```python
from build123d import *

# Parameters (mm, degrees)
F0_W     = 100.2733111382
F0_H     = 50.1366546378
F1_DEPTH = 50
F2_W     = 90.2733111382
F2_H     = 8.7347067715
F3_DEPTH = 50.001
F5_W     = 40.5144635588
F5_H     = 41.020902805
F6_DEPTH = 100.2743111382
F7_W     = 89.8914821446
F7_H     = 32.1583626792
F8_DEPTH = 50.001
F9_SCALE = 0.5


with BuildPart() as f1:
    # F0 (on Front) → F1 (new body)
    with BuildSketch(Plane.XZ):
        with Locations((-15.6993567944, 31.3960765488)):
            Rectangle(F0_W, F0_H)
    extrude(amount=F1_DEPTH)

    # F2 (on face) → F3 (cut, through all)
    with BuildSketch(Plane.XZ.offset(50)):
        with Locations((-15.6993567944, 47.097050482)):
            Rectangle(F2_W, F2_H)
    extrude(amount=-F3_DEPTH, mode=Mode.SUBTRACT)

    # F5 (on face) → F6 (cut, through all)
    with BuildSketch(Plane(origin=(-65.8360123634, 0, 0), x_dir=(0, -1, 0), z_dir=(-1, 0, 0))):
        with Locations((24.5618959889, 29.3703549542)):
            Rectangle(F5_W, F5_H)
    extrude(amount=-F6_DEPTH, mode=Mode.SUBTRACT)

    # F7 (on face) → F8 (cut, through all)
    with BuildSketch(Plane.XZ.offset(50)):
        with Locations((-16.0791818053, 22.4069305696)):
            Rectangle(F7_W, F7_H)
    extrude(amount=-F8_DEPTH, mode=Mode.SUBTRACT)


with BuildPart() as f1_1:
    # F9: moved
    add(f1.part.scale(F9_SCALE))


solid = f1_1.part
```
Design review of the part built by this model. Coordinates are the model's own, in mm. A direction names the side the tool comes from. Coordinates: 2 decimals unless noted, no trailing zeros. Order: outer loops, then holes, each group sorted by start corner. A loop starts at its lowest first (then second) coordinate and runs counter-clockwise, first axis right, second up.
1) Take a section at B-B, the plane x = -29. Give the boundary of the cut face in (y, z).
2) Take a section at A-A, the plane y = -9.25. Give the boundary of the cut face in (x, z).
3) For faces 1 (the flat face through (-8, 0, 20)), 2 (the flat face through (-8, -24, 21.365)), 3 (the flat face through (16, -12, 3.164)), 4 (the flat face through (16, -12, 4.43)), 5 (the flat face through (-8, -24, 19.243)), list the 3-axis set-ups (+Z, -Z, +X, -X, +Y, -Y) from which the entire face can be reached by the end or side of a thin tool; tool diameter is ignored.
4) Clearance check with flat-ended pins moving along their axes: pin 1 (10.5 mm diameter, centred on x = -6, z = 12.5, fed in from -Y); pin 2 (10 mm diameter, centred on x = -17.5, y = -12.5, fed in from -Z); pin 3 (10 mm diameter, centred on x = -2, y = -4.5, fed in from -Z). State where each tip first meets the part, or that it passes through.
5) Wall thickness on line 1 along Z through (x, y) = (-31, -18.25); line 2 along Z through (x, y) = (-29, -8.75); line 3 along Z through (x, y) = (0, -24): over which ranges is each line inside the solid? List them lowest first.
6) Mouldability with a two-part tool opening along Z and no side actions: class faces 6 (the flat face through (-8, -22.41, 20)), 7 (the flat face through (14.433, -14, 4)), 8 (the flat face through (-32, -12, 3.164)), 9 (the flat face through (-8, -12, 28.232)) as +Z half, -Z half, draft (parallel to the pull), parting line (faces both ways), or undercut.
7) Take a section at C-C, the plane z = 7.75. Give the boundary of the cut face in (x, y), and give its area (3 significant figures).
Returned:
1. outline: (-25, 19.24) - (-22.41, 19.24) - (-22.41, 21.36) - (-25, 21.36) - close; (-25, 25.73) - (0, 25.73) - (0, 28.23) - (-25, 28.23) - close; (-2.15, 19.24) - (0, 19.24) - (0, 21.36) - (-2.15, 21.36) - close
2. outline: (-32.92, 3.16) - (-30.51, 3.16) - (-30.51, 4.43) - (-32.92, 4.43) - close; (-32.92, 24.94) - (-30.42, 24.94) - (-30.42, 25.73) - (14.72, 25.73) - (14.72, 24.94) - (17.22, 24.94) - (17.22, 28.23) - (-32.92, 28.23) - close; (14.43, 3.16) - (17.22, 3.16) - (17.22, 4.43) - (14.43, 4.43) - close
3. face 1: +Z, -Z, +X, -X, +Y
3. face 2: +Y, -Y
3. face 3: -Z, +X, -X, +Y, -Y
3. face 4: +X, -X
3. face 5: -Z, +Y, -Y
4. pin 1: passes through
4. pin 2: stops at z = 25.73
4. pin 3: stops at z = 19.24
5. line 1: z = 3.16 to 4.43, 24.94 to 28.23
5. line 2: z = 25.73 to 28.23
5. line 3: z = 19.24 to 21.36, 25.73 to 28.23
6. face 6: undercut
6. face 7: draft
6. face 8: -Z half
6. face 9: +Z half
7. outline: (-32.92, -25) - (-30.51, -25) - (-30.51, -22.41) - (-32.92, -22.41) - close; (-32.92, -2.15) - (-30.51, -2.15) - (-30.51, 0) - (-32.92, 0) - close; (14.43, -25) - (17.22, -25) - (17.22, -22.41) - (14.43, -22.41) - close; (14.43, -2.15) - (17.22, -2.15) - (17.22, 0) - (14.43, 0) - close
7. area: 24.6 mm2
